from build123d import *

# Parameters (mm, degrees)
BOSS_EXTRUDE2_DEPTH = 4.7625
CUT_EXTRUDE1_REACH  = 553.521
FILLET1_R           = 25.4
SKETCH3_W           = 63.5
SKETCH3_H           = 4.7625
SKETCH3_H_2         = 6.35
SKETCH3_W_2         = 12.7
SKETCH3_H_3         = 25.4
CUT_EXTRUDE2_DEPTH  = 552.520896165
SKETCH4_W           = 9.144
SKETCH4_H           = 12.954
SKETCH4_R           = 1.7145
SKETCH4_R_2         = 6.35
CUT_EXTRUDE3_DEPTH  = 552.520896165


with BuildPart() as part:
    # Sketch1 → Boss-Extrude2 (new body)
    with BuildSketch(Plane.XY):
        Polygon((-95.25, 450.939427751), (95.25, 450.939427751), (317.5, 65.991135768), (279.4, 0), (-279.4, 0), (-317.5, 65.991135768), align=None)
    extrude(amount=BOSS_EXTRUDE2_DEPTH)

    # Sketch2 → Cut-Extrude1 (cut, up to next)
    with BuildSketch(Plane.XY.offset(4.7625), mode=Mode.PRIVATE) as cut_extrude1_sk1:
        Polygon((-92.808632673, 378.968), (92.808632673, 378.968), (273.505909488, 65.991135768), (257.402954744, 38.1), (-257.402954744, 38.1), (-273.505909488, 65.991135768), align=None)
    cut_extrude1_tool1 = extrude(cut_extrude1_sk1.sketch, amount=-CUT_EXTRUDE1_REACH, mode=Mode.PRIVATE) & part.part
    add(cut_extrude1_tool1.solids().sort_by_distance((0, 180.212896, 4.7625))[0], mode=Mode.SUBTRACT)

    # Fillet1
    fillet1_edges = [part.edges().sort_by_distance(p)[0] for p in [
        (-273.505909488, 65.991135768, 2.38125),
        (-92.808632673, 378.968, 2.38125),
        (92.808632673, 378.968, 2.38125),
        (273.505909488, 65.991135768, 2.38125),
        (257.402954744, 38.1, 2.38125),
        (-257.402954744, 38.1, 2.38125),
    ]]
    fillet(fillet1_edges, radius=FILLET1_R)

    # Sketch3 → Cut-Extrude2 (cut, through all)
    with BuildSketch(Plane.XY.offset(4.7625)):
        with Locations((-222.25, 2.38125)):
            Rectangle(SKETCH3_W, SKETCH3_H)
        with Locations((-114.3, 2.38125)):
            Rectangle(SKETCH3_W, SKETCH3_H)
        with Locations((0, 3.175)):
            Rectangle(SKETCH3_W, SKETCH3_H_2)
        Polygon((-199.263, 270.783627103), (-195.138554014, 268.402377103), (-230.698554014, 206.810650386), (-234.823, 209.191900386), align=None)
        Polygon((-269.875, 148.480055479), (-265.750554014, 146.098805479), (-297.500554014, 91.106192339), (-301.625, 93.487442339), align=None)
        Polygon((-309.5625, 52.242982483), (-305.438054014, 54.624232483), (-283.213054014, 16.129403285), (-287.3375, 13.748153285), align=None)
        Polygon((287.3375, 13.748153285), (309.5625, 52.242982483), (305.438054014, 54.624232483), (283.213054014, 16.129403285), align=None)
        Polygon((301.625, 93.487442339), (269.875, 148.480055479), (265.750554014, 146.098805479), (297.500554014, 91.106192339), align=None)
        Polygon((234.823, 209.191900386), (199.263, 270.783627103), (195.138554014, 268.402377103), (230.698554014, 206.810650386), align=None)
        with Locations((114.3, 2.38125)):
            Rectangle(SKETCH3_W, SKETCH3_H)
        with Locations((222.25, 2.38125)):
            Rectangle(SKETCH3_W, SKETCH3_H)
        with Locations((-25.4, 438.239427751)):
            Rectangle(SKETCH3_W_2, SKETCH3_H_3)
        with Locations((25.4, 438.239427751)):
            Rectangle(SKETCH3_W_2, SKETCH3_H_3)
    extrude(amount=-CUT_EXTRUDE2_DEPTH, mode=Mode.SUBTRACT)

    # Sketch4 → Cut-Extrude3 (cut, through all)
    with BuildSketch(Plane.XY.offset(4.7625)):
        Polygon((-239.352506919, 175.438564268), (-250.571, 181.915564268), (-255.143, 173.996627976), (-243.924506919, 167.519627976), align=None)
        with Locations((-164.592, 6.477)):
            Rectangle(SKETCH4_W, SKETCH4_H)
        with Locations((164.592, 6.477)):
            Rectangle(SKETCH4_W, SKETCH4_H)
        Polygon((250.571, 181.915564268), (239.352506919, 175.438564268), (243.924506919, 167.519627976), (255.143, 173.996627976), align=None)
        with Locations((-12.7, 29.845)):
            Circle(SKETCH4_R)
        with Locations((12.7, 29.845)):
            Circle(SKETCH4_R)
        with Locations((63.5, 400.139427751)):
            Circle(SKETCH4_R_2)
        with Locations((-63.5, 400.139427751)):
            Circle(SKETCH4_R_2)
    extrude(amount=-CUT_EXTRUDE3_DEPTH, mode=Mode.SUBTRACT)


solid = part.part
The listing builds one solid part. Answer for the finished solid, in the listing's coordinates (mm). A direction names the side the tool comes from. Coordinates: 2 decimals unless noted, no trailing zeros. Write each loop counter-clockwise with the first axis right and the second up, starting at its lowest first coordinate (ties: lowest second). Pieces come first, ordered by that corner, then holes. Notation, with made-up numbers: M 89.5,-16 L 101.5,-16 A36 cw 101.5,22 Z; hole C 80.5,-39.5 d1. An arc over 180 degrees is marked long. Put each result on its own line as item: value. Start each with the question number.
1. A cutting plane is placed at A-A on x = 63.5. Write down the section's boundary in (y, z), then the cut area to 3 significant figures.
2. A cutting plane is placed at C-C on z = 2.75. Count the separate pieces of the cut face and the enclosed holes in it, then the cut area to 3 significant figures.
3. Consider line 1 (Y direction, x = 63.5, z = 3.1); line 2 (Y direction, x = 12.7, z = 1.35); line 3 (Y direction, x = -26.5, z = 3.95). Determine where each line is inside the solid, lowest interval first. Write a range as from..to.
4. Which of the six approach directions +Z, -Z, +X, -X, +Y, -Y give full straight-line access (tool end or side, diameter ignored) to faces 1 (the flat face through (-242.81, 195.36, 2.35)), 2 (the cylindrical face through (-90.68, 375.66, 2.35))?
5. A cutting plane is placed at D-D on y = 189.5. Write down the section's boundary in (x, z), then the cut area to 3 significant figures.
6. Flat-ended cylindrical pins translate along their axes: P1, Ø1.4, axis at x = -213, z = 3, coming from the -Y side; P2, Ø1.4, axis at x = -26, z = 3.5, coming from the +Y side; P3, Ø1.4, axis at y = 8.5, z = 2, coming from the +X side. Find the tip coordinate at first contact, or state that the pin passes through.
7. For a pull along X with two mould halves and no side action, classify faces 3 (the flat face through (262.406, 161.417, 2.348)), 4 (the flat face through (-262.61, 161.06, 2.35)), 5 (the cylindrical face through (-64.88, 393.94, 2.41)) as pulls with the +X half, pulls with the -X half, needs draft (parallel to the pull), parting line crosses it, or undercut.
8. A cutting plane is placed at B-B on y = 235. Write down the section's boundary in (x, z), then the cut area to 3 significant figures.
Resolved:
1. outline: M 0,0 L 38.1,0 L 38.1,4.76 L 0,4.76 Z; M 378.97,0 L 393.79,0 L 393.79,4.76 L 378.97,4.76 Z; M 406.49,0 L 450.94,0 L 450.94,4.76 L 406.49,4.76 Z
1. area: 464 mm2
2. separate pieces: 1
2. enclosed holes: 5
2. area: 64,300 mm2
3. line 1: y = 0..38.1, 378.97..393.79, 406.49..450.94
3. line 2: y = 6.35..28.13, 31.56..38.1, 378.97..450.94
3. line 3: y = 6.35..38.1, 378.97..425.54
4. face 1: +Z, -Z, -X, +Y
4. face 2: +Z, -Z
5. outline: M -246.19,0 L -202.2,0 L -202.2,4.76 L -246.19,4.76 Z; M 202.2,0 L 246.19,0 L 246.19,4.76 L 202.2,4.76 Z
5. area: 419 mm2
6. P1: stops at y = 4.76
6. P2: stops at y = 425.54
6. P3: stops at x = 284.71
7. face 3: pulls with the +X half
7. face 4: pulls with the -X half
7. face 5: undercut
8. outline: M -214.42,0 L -175.93,0 L -175.93,4.76 L -214.42,4.76 Z; M 175.93,0 L 214.42,0 L 214.42,4.76 L 175.93,4.76 Z
8. area: 367 mm2
